The listing builds one solid part. Answer for the finished solid, in the listing's coordinates (mm). Face numbers are marked on the shaded views. A direction names the side the tool comes from. Round coordinates to 2 decimals unless told otherwise and drop trailing zeros. Write each loop counter-clockwise with the first axis right and the second up, starting at its lowest first coordinate (ties: lowest second). Pieces come first, ordered by that corner, then holes.
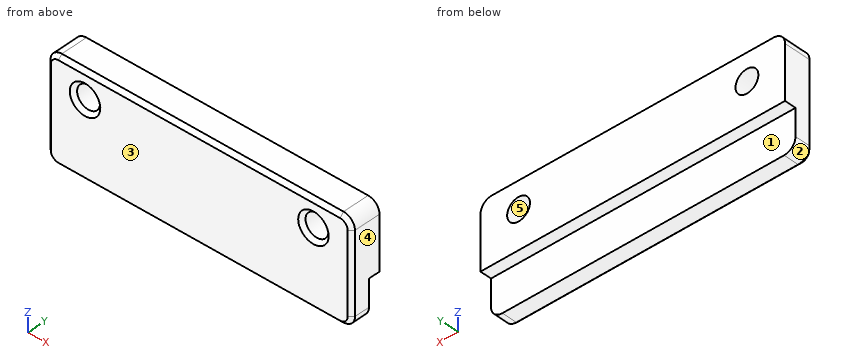
from build123d import *

# Parameters (mm, degrees)
SKETCH1_R           = 3
BOSS_EXTRUDE1_DEPTH = 8
SKETCH2_W           = 10
SKETCH2_H           = 3
CUT_EXTRUDE1_DEPTH  = 83.849260709
FILLET1_R           = 3
CHAMFER1_SIZE       = 1


with BuildPart() as part:
    # Sketch1 → Boss-Extrude1 (new body)
    with BuildSketch(Plane(origin=(0, 0, 0), x_dir=(1, 0, 0), z_dir=(0, 1, 0))):
        Polygon((-40, 20), (40, 20), (40, -7), (30, -7), (-40, -7), align=None)
        with Locations(Location((30, 0, 0), (0, 0, 270))):
            Circle(SKETCH1_R, mode=Mode.SUBTRACT)
        with Locations(Location((-30, 0, 0), (0, 0, 270))):
            Circle(SKETCH1_R, mode=Mode.SUBTRACT)
    extrude(amount=BOSS_EXTRUDE1_DEPTH)

    # Sketch2 → Cut-Extrude1 (cut, through all)
    with BuildSketch(Plane(origin=(40, 0, 0), x_dir=(0, 0, -1), z_dir=(1, 0, 0))):
        with Locations((15, 6.5)):
            Rectangle(SKETCH2_W, SKETCH2_H)
    extrude(amount=-CUT_EXTRUDE1_DEPTH, mode=Mode.SUBTRACT)

    # Fillet1
    fillet1_edges = [part.edges().sort_by_distance(p)[0] for p in [
        (-40, 4, 7),
        (40, 4, 7),
        (-40, 2.5, -20),
        (40, 2.5, -20),
    ]]
    fillet(fillet1_edges, radius=FILLET1_R)

    # Chamfer1
    chamfer1_edges = [part.edges().sort_by_distance(p)[0] for p in [
        (-40, 0, -6.5),
        (0, 0, 7),
        (0, 0, -20),
        (40, 0, -6.5),
        (39.121320344, 0, -19.121320344),
        (39.121320344, 0, 6.121320344),
        (-39.121320344, 0, 6.121320344),
        (-39.121320344, 0, -19.121320344),
        (-30, 0, -3),
        (30, 0, -3),
    ]]
    chamfer(chamfer1_edges, length=CHAMFER1_SIZE)


solid = part.part
1. Section B-B on x = -30 is taken. Determine the outline of the cut face in (y, z), plus the area to 3 significant figures.
Geometry says:
outline: (0, -19) - (1, -20) - (5, -20) - (5, -10) - (8, -10) - (8, -3) - (1, -3) - (0, -4) - close; (0, 4) - (1, 3) - (8, 3) - (8, 7) - (1, 7) - (0, 6) - close
area: 136 mm2
2. Section D-D on z = -13 is taken. Determine the outline of the cut face in (x, y), plus the area to 3 significant figures.
Geometry says:
outline: (-40, 1) - (-39, 0) - (39, 0) - (40, 1) - (40, 5) - (-40, 5) - close
area: 399 mm2
3. Straight lines are drawn through the part: line 1 along X through (y, z) = (4.75, 0); line 2 along X through (y, z) = (5, -0.75); line 3 along Y through (x, z) = (32, -18.5). For each, find the intervals that lie inside material, in ascending order.
Geometry says:
line 1: x = -40 to -33, -27 to 27, 33 to 40
line 2: x = -40 to -32.9, -27.1 to 27.1, 32.9 to 40
line 3: y = 0 to 5
4. Section C-C on y = 5.75 is taken. Determine the outline of the cut face in (x, z).
Geometry says:
outline: (-40, -10) - (40, -10) - (40, 4) arc R3 ccw to (37, 7) - (-37, 7) arc R3 ccw to (-40, 4) - close; hole circle Ø6 at (-30, 0); hole circle Ø6 at (30, 0)
5. Section A-A on z = 0 is taken. Determine the outline of the cut face in (x, y).
Geometry says:
outline: (-40, 1) - (-39, 0) - (-34, 0) - (-33, 1) - (-33, 8) - (-40, 8) - close; (-27, 1) - (-26, 0) - (26, 0) - (27, 1) - (27, 8) - (-27, 8) - close; (33, 1) - (34, 0) - (39, 0) - (40, 1) - (40, 8) - (33, 8) - close
6. A tool of negligible diameter and unlimited length cuts with its end or side. For the marked faces 1 and 2, from which of +Z, -Z, +X, -X, +Y, -Y can it reach the whole face along a straight path? Write none if from no direction.
Geometry says:
face 1: -Z, +X, -X, +Y
face 2: -Z, -X, +Y, -Y
7. For a pull along X with two mould halves and no side action, classify the marked faces 3, 4 and 5 as released by +X, released by -X, zero draft, split by the parting line, or undercut.
Geometry says:
face 3: zero draft
face 4: released by +X
face 5: undercut
8. Given pin 1 (0.9 mm diameter, centred on x = 7.5, y = 6, fed in from -Z); pin 2 (3 mm diameter, centred on x = 11.5, z = -16.5, fed in from +Y); pin 3 (7 mm diameter, centred on x = -30, z = 0, fed in from -Y), each flat-ended and moving along its own axis, determine where each tip first touches the part or whether it passes through.
Geometry says:
pin 1: stops at z = -10
pin 2: stops at y = 5
pin 3: stops at y = 0.5
